The drawing under review shows one solid part. Ordinate dimensions are in mm from its lowest x, y, z. A direction names the side the tool comes from. Round coordinates to 2 decimals unless told otherwise and drop trailing zeros. Order: outer loops, then holes, each group sorted by start corner. A loop starts at its lowest first (then second) coordinate and runs counter-clockwise, first axis right, second up. Notation, with made-up numbers: M -24,-26 L -17,-26 A9 ccw -17,-13 Z; hole C 35,47.25 d8. An arc over 180 degrees is marked long. Answer as a JSON object with one key per item and string values. Group by question number.
1. Add section C-C on z = 76.5. State the section outline as (x, y) points, and give its area (4 significant figures).
2. Clearance check with a flat-ended pin moving along its axis: P1, Ø3, axis at y = 143.5, z = 48.5, coming from the +X side. State where the tip first meets the part, or that it passes through.
3. To check wall thickness, follow probe 1 along Z at (x, y) = (46, 112.5); probe 2 along X at (y, z) = (104.5, 40.5); probe 3 along Z at (x, y) = (9, 87.5). State the ranges of each line that lie inside material, in increasing order. Write a range as [from, to].
4. Add section A-A on y = 49.5. State the section outline as (x, z) points.
5. Machinability: for the marked faces 1 and 2, which of the approach directions +Z, -Z, +X, -X, +Y, -Y give a long, thin tool a straight path to every point of the face, cutting with its end or side? Answer none if there is none.
6. Add section B-B on x = 19. State the section outline as (y, z) points.
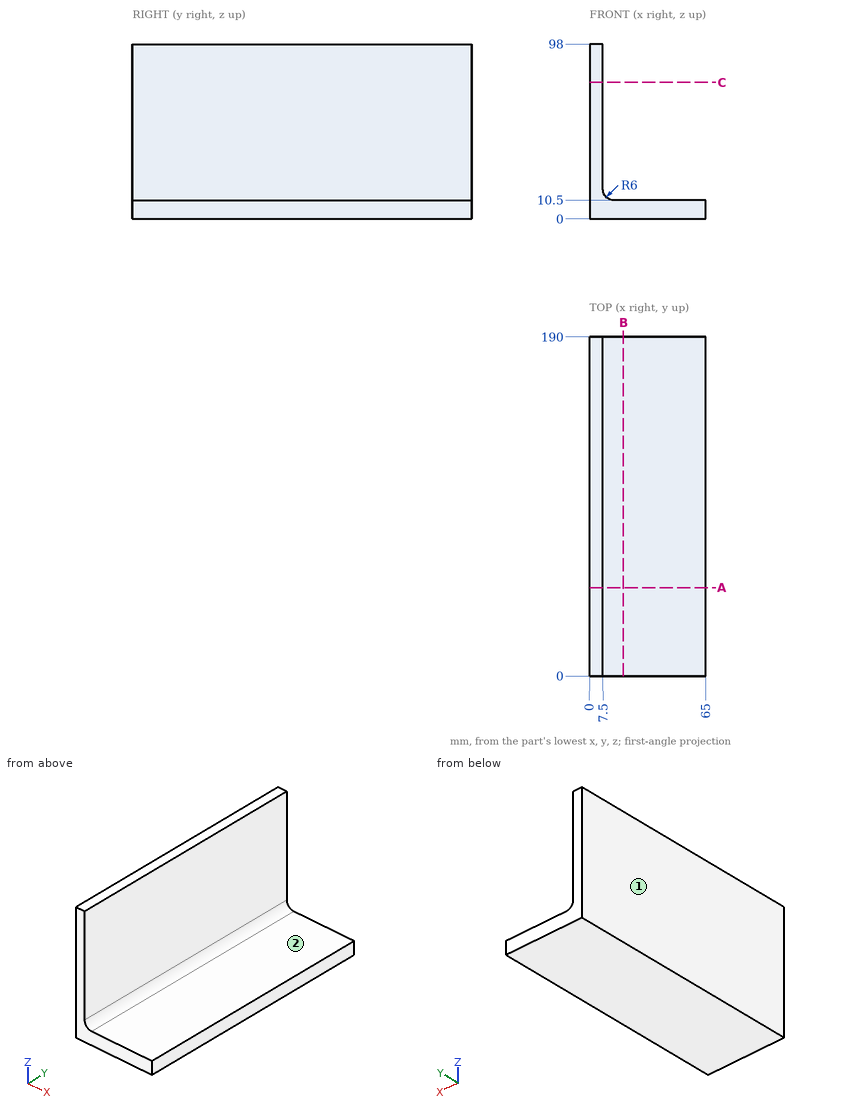
Recorded:
{
 "1": {"outline": "M 0,0 L 7.5,0 L 7.5,190 L 0,190 Z", "area": "1,425 mm²"},
 "2": {"P1": "stops at x = 7.5"},
 "3": {"probe 1": "z = [0, 10.5]", "probe 2": "x = [0, 7.5]", "probe 3": "z = [0, 12.53]"},
 "4": {"outline": "M 0,0 L 65,0 L 65,10.5 L 13.5,10.5 A6 cw 7.5,16.5 L 7.5,98 L 0,98 Z"},
 "5": {"face 1": "+Z, -Z, -X, +Y, -Y", "face 2": "+Z, +X, +Y, -Y"},
 "6": {"outline": "M 0,0 L 190,0 L 190,10.5 L 0,10.5 Z"}
}
